Verification items for this drawing (mm, ordinates from the low corner). A direction names the side the tool comes from. Coordinates: 2 decimals unless noted, no trailing zeros. Write each loop counter-clockwise with the first axis right and the second up, starting at its lowest first coordinate (ties: lowest second). Pieces come first, ordered by that corner, then holes.
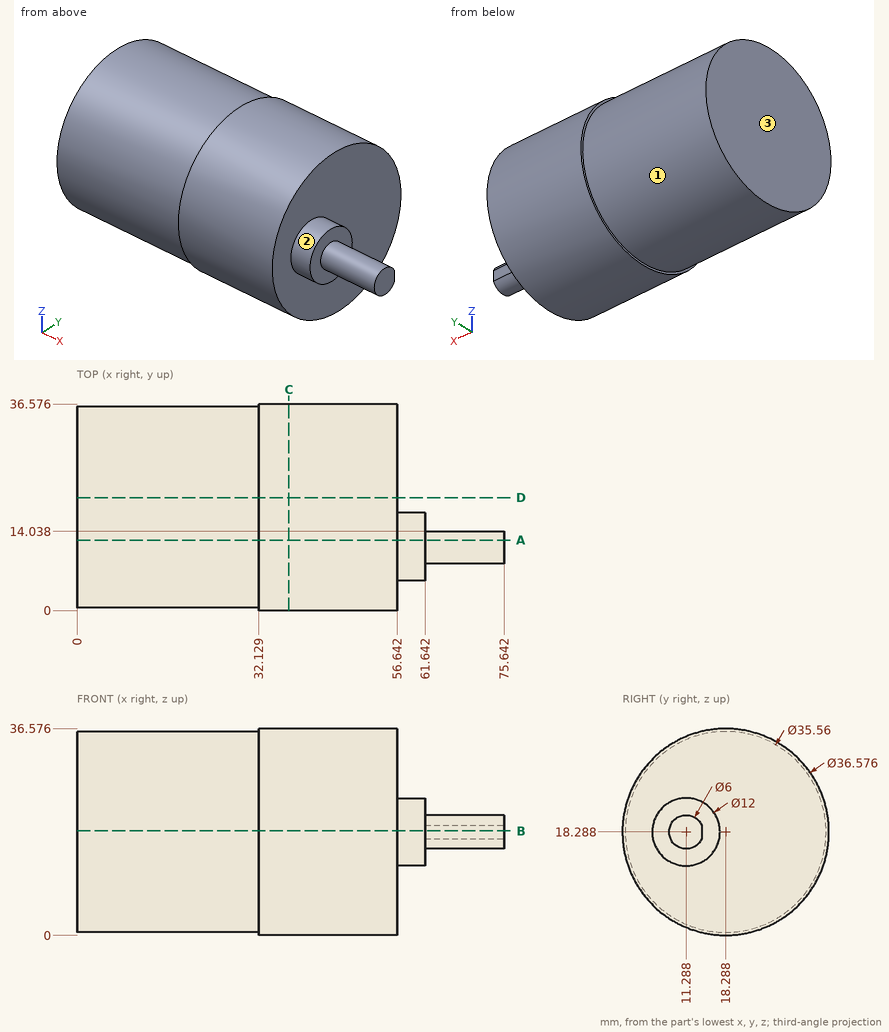
1. Sectioned sample at B-B, the plane z = 18.5. Record the boundary of the cut face in (x, y) (1 decimal), and give its area (3 significant figures).
Computed values:
outline: (0, 0.5) - (32.1, 0.5) - (32.1, 0) - (56.6, 0) - (56.6, 5.3) - (61.6, 5.3) - (61.6, 8.3) - (75.6, 8.3) - (75.6, 14) - (61.6, 14) - (61.6, 17.3) - (56.6, 17.3) - (56.6, 36.6) - (32.1, 36.6) - (32.1, 36.1) - (0, 36.1) - close
area: 2,180 mm2
2. Gauge pin test, flat ends, axial feed: pin 1 Ø3 at (x, y) = (52.5, 11) entering from -Z; pin 2 Ø1.9 at (x, z) = (71.5, 18) entering from +Y; pin 3 Ø8 at (x, z) = (31.5, 27) entering from -Y. Record the tip position at first contact, or that the pin passes through.
Computed values:
pin 1: stops at z = 0.94
pin 2: stops at y = 14.04
pin 3: stops at y = 0.63
3. Thickness scan on line 1 along X through (y, z) = (24.5, 20); line 2 along Y through (x, z) = (37, 10) (1 decimal); line 3 along Z through (x, y) = (14, 5.5) (1 decimal). Record the ranges inside material, lowest first.
Computed values:
line 1: x = 0 to 56.64
line 2: y = 2 to 34.6
line 3: z = 5.9 to 30.6
4. Sectioned sample at C-C, the plane x = 37.5. Record the boundary of the cut face in (y, z).
Computed values:
outline: circle Ø36.58 at (18.29, 18.29)
5. Sectioned sample at D-D, the plane y = 20. Record the boundary of the cut face in (x, z) (1 decimal).
Computed values:
outline: (0, 0.6) - (32.1, 0.6) - (32.1, 0.1) - (56.6, 0.1) - (56.6, 36.5) - (32.1, 36.5) - (32.1, 36) - (0, 36) - close
6. Access from +Z, -Z, +X, -X, +Y, -Y to the whole of each face (thin tool, end or side, straight path). Record for the marked faces 1, 2 and 3.
Computed values:
face 1: -X
face 2: +X
face 3: +Z, -Z, -X, +Y, -Y
7. Sectioned sample at A-A, the plane y = 12.5. Record the boundary of the cut face in (x, z), and give its area (3 significant figures).
Computed values:
outline: (0, 1.48) - (32.13, 1.48) - (32.13, 0.94) - (56.64, 0.94) - (56.64, 12.41) - (61.64, 12.41) - (61.64, 15.54) - (75.64, 15.54) - (75.64, 21.03) - (61.64, 21.03) - (61.64, 24.16) - (56.64, 24.16) - (56.64, 35.64) - (32.13, 35.64) - (32.13, 35.1) - (0, 35.1) - close
area: 2,070 mm2
